```python
from build123d import *

# Parameters (mm, degrees)
PAD_DEPTH       = 14
POCKET_DEPTH    = 12.4
SKETCH002_R     = 1.5
PAD001_DEPTH    = 3.2
SKETCH003_R     = 1.05
PAD002_DEPTH    = 1.6
POCKET001_DEPTH = 0.8
POCKET003_DEPTH = 1.6
POCKET008_DEPTH = 1.6


with BuildPart() as part:
    # Sketch → Pad (new body)
    with BuildSketch(Plane.XY):
        with BuildLine():
            Line((-19.6, 18.1), (-19.6, -18.1))
            ThreePointArc((-19.6, -18.1), (-19.16066, -19.16066), (-18.1, -19.6))
            Line((-18.1, -19.6), (18.1, -19.6))
            ThreePointArc((18.1, -19.6), (19.16066, -19.16066), (19.6, -18.1))
            Line((19.6, -18.1), (19.6, 18.1))
            ThreePointArc((19.6, 18.1), (19.16066, 19.16066), (18.1, 19.6))
            Line((18.1, 19.6), (-18.1, 19.6))
            ThreePointArc((-18.1, 19.6), (-19.16066, 19.16066), (-19.6, 18.1))
        make_face()
    extrude(amount=PAD_DEPTH)

    # Sketch001 (on Face10 of Pad) → Pocket (cut)
    with BuildSketch(Plane.XY.offset(14)):
        with BuildLine():
            Line((-18.8, 17.3), (-18.8, -17.3))
            ThreePointArc((-18.8, -17.3), (-18.36066, -18.36066), (-17.3, -18.8))
            Line((-17.3, -18.8), (17.3, -18.8))
            ThreePointArc((17.3, -18.8), (18.36066, -18.36066), (18.8, -17.3))
            Line((18.8, -17.3), (18.8, 17.3))
            ThreePointArc((18.8, 17.3), (18.36066, 18.36066), (17.3, 18.8))
            Line((17.3, 18.8), (-17.3, 18.8))
            ThreePointArc((-17.3, 18.8), (-18.36066, 18.36066), (-18.8, 17.3))
        make_face()
    extrude(amount=-POCKET_DEPTH, mode=Mode.SUBTRACT)

    # Sketch002 (on Face19 of Pocket) → Pad001 (join)
    with BuildSketch(Plane.XY.offset(1.6)):
        with Locations((-15, 15)):
            Circle(SKETCH002_R)
        with Locations((15, 15)):
            Circle(SKETCH002_R)
        with Locations((-15, -15)):
            Circle(SKETCH002_R)
        with Locations((15, -15)):
            Circle(SKETCH002_R)
    extrude(amount=PAD001_DEPTH)

    # Sketch003 (on Face27 of Pad001) → Pad002 (join)
    with BuildSketch(Plane.XY.offset(4.8)):
        with Locations((-15, 15)):
            Circle(SKETCH003_R)
        with Locations((15, 15)):
            Circle(SKETCH003_R)
        with Locations((-15, -15)):
            Circle(SKETCH003_R)
        with Locations((15, -15)):
            Circle(SKETCH003_R)
    extrude(amount=PAD002_DEPTH)

    # Sketch004 (on Face7 of Pad002) → Pocket001 (cut)
    with BuildSketch(Plane.XZ.offset(19.6)):
        with BuildLine():
            Line((-4.5, 8.575), (-4.5, 7.375))
            ThreePointArc((-4.5, 7.375), (-4.207107, 6.667893), (-3.5, 6.375))
            Line((-3.5, 6.375), (3.5, 6.375))
            ThreePointArc((3.5, 6.375), (4.207107, 6.667893), (4.5, 7.375))
            Line((4.5, 7.375), (4.5, 8.575))
            ThreePointArc((4.5, 8.575), (4.207107, 9.282107), (3.5, 9.575))
            Line((3.5, 9.575), (-3.5, 9.575))
            ThreePointArc((-3.5, 9.575), (-4.207107, 9.282107), (-4.5, 8.575))
        make_face()
    extrude(amount=-POCKET001_DEPTH, mode=Mode.SUBTRACT)

    # Sketch009 (on Face4 of Pocket001) → Pocket003 (cut)
    with BuildSketch(Plane(origin=(0, 0, 0), x_dir=(1, 0, 0), z_dir=(0, 0, -1))):
        with BuildLine():
            Line((-6.495191, 3.75), (-3.307189, 3.75))
            ThreePointArc((3.307189, 3.75), (0, 5), (-3.307189, 3.75))
            Line((3.307189, 3.75), (6.495191, 3.75))
            ThreePointArc((6.495191, -3.75), (7.5, 0), (6.495191, 3.75))
            Line((3.307189, -3.75), (6.495191, -3.75))
            ThreePointArc((-3.307189, -3.75), (0, -5), (3.307189, -3.75))
            Line((-6.495191, -3.75), (-3.307189, -3.75))
            ThreePointArc((-6.495191, 3.75), (-7.5, 0), (-6.495191, -3.75))
        make_face()
    extrude(amount=-POCKET003_DEPTH, mode=Mode.SUBTRACT)

    # Sketch029 (on Face4 of Pocket003) → Pocket008 (cut)
    with BuildSketch(Plane(origin=(0, 0, 0), x_dir=(1, 0, 0), z_dir=(0, 0, -1))):
        with BuildLine():
            Line((-10, 17.5), (10, 17.5))
            ThreePointArc((10.4, 17.1), (10.282843, 17.382843), (10, 17.5))
            Line((10.4, 17.1), (10.4, 16.4))
            ThreePointArc((10, 16), (10.282843, 16.117157), (10.4, 16.4))
            Line((10, 16), (-10, 16))
            ThreePointArc((-10.4, 16.4), (-10.282843, 16.117157), (-10, 16))
            Line((-10.4, 16.4), (-10.4, 17.1))
            ThreePointArc((-10, 17.5), (-10.282843, 17.382843), (-10.4, 17.1))
        make_face()
        with BuildLine():
            Line((-10, -16), (10, -16))
            ThreePointArc((10.4, -16.4), (10.282843, -16.117157), (10, -16))
            Line((10.4, -16.4), (10.4, -17.1))
            ThreePointArc((10, -17.5), (10.282843, -17.382843), (10.4, -17.1))
            Line((10, -17.5), (-10, -17.5))
            ThreePointArc((-10.4, -17.1), (-10.282843, -17.382843), (-10, -17.5))
            Line((-10.4, -17.1), (-10.4, -16.4))
            ThreePointArc((-10, -16), (-10.282843, -16.117157), (-10.4, -16.4))
        make_face()
    extrude(amount=-POCKET008_DEPTH, mode=Mode.SUBTRACT)


with BuildPart() as part_1:
    # Body placement: moved
    add(part.part.moved(Location((0, 0, -0.8))))


solid = part_1.part
```
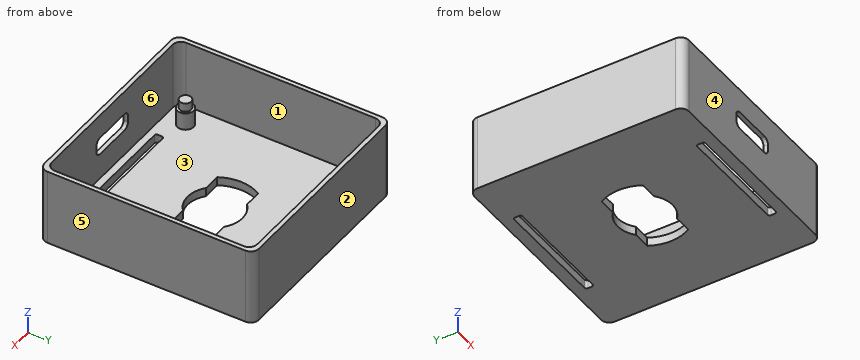
Work out the finished part from the listing and answer in its coordinate system (mm). Face numbers are marked on the shaded views. A direction names the side the tool comes from. Round coordinates to 2 decimals unless told otherwise and drop trailing zeros. Loops run counter-clockwise (first coordinate to the right, second up) from the corner with the lowest first, then second, coordinate; pieces in that order, holes last.
(1) For the marked faces 1 and 2, determine the directions among +Z, -Z, +X, -X, +Y, -Y from which every point of the face is accessible in a straight line to the end or side of a thin tool.
Computed values:
face 1: +Z
face 2: +Z, -Z, +X, -X, +Y
(2) The part is cut by section C-C, the plane y = 15. Give the vertices of the cut face in (x, z).
Computed values:
outline: (-19.6, -0.8) - (19.6, -0.8) - (19.6, 13.2) - (18.8, 13.2) - (18.8, 0.8) - (16.5, 0.8) - (16.5, 4) - (16.05, 4) - (16.05, 5.6) - (13.95, 5.6) - (13.95, 4) - (13.5, 4) - (13.5, 0.8) - (-13.5, 0.8) - (-13.5, 4) - (-13.95, 4) - (-13.95, 5.6) - (-16.05, 5.6) - (-16.05, 4) - (-16.5, 4) - (-16.5, 0.8) - (-18.8, 0.8) - (-18.8, 13.2) - (-19.6, 13.2) - close
(3) Each of these flat-tipped pins is pushed along its axis until it touches: P1, Ø11.5, axis at x = 2, y = -5, coming from the +Z side; P2, Ø1.1, axis at x = 14.5, y = -15.5, coming from the +Z side. Where does it stop, or does it pass through?
Computed values:
P1: stops at z = 0.8
P2: stops at z = 5.6
(4) The mould has two halves that part along Y. Classify the marked faces 3, 4, 5 and 6: pulls with the +Y half, pulls with the -Y half, needs draft (parallel to the pull), parting line crosses it, or undercut.
Computed values:
face 3: undercut
face 4: pulls with the -Y half
face 5: needs draft
face 6: undercut
(5) The part is cut by section A-A, the plane y = -11. Give the vertices of the cut face in (x, z), and give its area (3 significant figures).
Computed values:
outline: (-19.6, -0.8) - (19.6, -0.8) - (19.6, 13.2) - (18.8, 13.2) - (18.8, 0.8) - (-18.8, 0.8) - (-18.8, 13.2) - (-19.6, 13.2) - close
area: 82.6 mm2
(6) Find the intervals of material crossed by L1, parallel to X at y = -3.5, z = 4.5; L2, parallel to X at y = -14.5, z = 3.5, in increasing order.
Computed values:
L1: x = -19.6 to -18.8, 18.8 to 19.6
L2: x = -19.6 to -18.8, -16.41 to -13.59, 13.59 to 16.41, 18.8 to 19.6
